```python
from build123d import *

# Parameters (mm, degrees)
MODEL_R             = 1.55
BOSS_EXTRUDE1_DEPTH = 3


with BuildPart() as part:
    # Model → Boss-Extrude1 (new body)
    with BuildSketch(Plane.XY):
        with BuildLine():
            Line((0, 108.6), (0, 5))
            ThreePointArc((0, 5), (1.464466094, 1.464466094), (5, 0))
            Line((5, 0), (365.775, 0))
            ThreePointArc((365.775, 0), (369.310533906, 1.464466094), (370.775, 5))
            Line((370.775, 5), (370.775, 108.6))
            ThreePointArc((370.775, 108.6), (369.310533906, 112.135533906), (365.775, 113.6))
            Line((365.775, 113.6), (5, 113.6))
            ThreePointArc((5, 113.6), (1.464466094, 112.135533906), (0, 108.6))
        make_face()
        with Locations((195.3875, 109.1)):
            Circle(MODEL_R, mode=Mode.SUBTRACT)
        with Locations((175.3875, 109.1)):
            Circle(MODEL_R, mode=Mode.SUBTRACT)
        with Locations((85.3875, 107.6)):
            Circle(MODEL_R, mode=Mode.SUBTRACT)
        with Locations((285.3875, 107.6)):
            Circle(MODEL_R, mode=Mode.SUBTRACT)
        with Locations((85.3875, 6)):
            Circle(MODEL_R, mode=Mode.SUBTRACT)
        with Locations((185.3875, 6)):
            Circle(MODEL_R, mode=Mode.SUBTRACT)
        with Locations((285.3875, 6)):
            Circle(MODEL_R, mode=Mode.SUBTRACT)
        Polygon((9, 9), (361.775, 9), (361.775, 104.6), (190.3875, 104.6), (190.3875, 106.6), (180.3875, 106.6), (180.3875, 104.6), (9, 104.6), align=None, mode=Mode.SUBTRACT)
        Polygon((365.947431604, 110.609548911), (367.784548911, 108.772431604), (367.112117307, 106.262882693), (364.602568396, 105.590451089), (362.765451089, 107.427568396), (363.437882693, 109.937117307), align=None, mode=Mode.SUBTRACT)
        Polygon((4.827568396, 110.609548911), (2.990451089, 108.772431604), (3.662882693, 106.262882693), (6.172431604, 105.590451089), (8.009548911, 107.427568396), (7.337117307, 109.937117307), align=None, mode=Mode.SUBTRACT)
        Polygon((365.947431604, 2.990451089), (367.784548911, 4.827568396), (367.112117307, 7.337117307), (364.602568396, 8.009548911), (362.765451089, 6.172431604), (363.437882693, 3.662882693), align=None, mode=Mode.SUBTRACT)
        Polygon((126.799038106, 2.25), (124.200961894, 2.25), (122.901923789, 4.5), (124.200961894, 6.75), (126.799038106, 6.75), (128.098076211, 4.5), align=None, mode=Mode.SUBTRACT)
        Polygon((4.827568396, 2.990451089), (2.990451089, 4.827568396), (3.662882693, 7.337117307), (6.172431604, 8.009548911), (8.009548911, 6.172431604), (7.337117307, 3.662882693), align=None, mode=Mode.SUBTRACT)
        Polygon((126.799038106, 111.35), (124.200961894, 111.35), (122.901923789, 109.1), (124.200961894, 106.85), (126.799038106, 106.85), (128.098076211, 109.1), align=None, mode=Mode.SUBTRACT)
        Polygon((243.975961894, 2.25), (246.574038106, 2.25), (247.873076211, 4.5), (246.574038106, 6.75), (243.975961894, 6.75), (242.676923789, 4.5), align=None, mode=Mode.SUBTRACT)
        Polygon((243.975961894, 111.35), (246.574038106, 111.35), (247.873076211, 109.1), (246.574038106, 106.85), (243.975961894, 106.85), (242.676923789, 109.1), align=None, mode=Mode.SUBTRACT)
    extrude(amount=BOSS_EXTRUDE1_DEPTH)


solid = part.part
```
Model file for the job. Use its own axes, mm. Coordinates: 2 decimals unless noted, no trailing zeros. Write each loop counter-clockwise with the first axis right and the second up, starting at its lowest first coordinate (ties: lowest second). Pieces come first, ordered by that corner, then holes. Notation, with made-up numbers: (-8.75, 68.25) - (46.25, 68.25) arc R14 cw to (46.25, 77.25) - close; hole circle Ø10 at (28.5, 3). An arc over 180 degrees is marked (long way). One line per item, written item: value. Start each with the question number.
1. Slice it at B-B (z = 0.95). Count the separate pieces of the cut face and the enclosed holes in it, plus the area to 3 significant figures.
2. Probe line 1 (Y direction, x = 126, z = 2.4); line 2 (Y direction, x = 137, z = 1.85); line 3 (X direction, y = 37, z = 0.85) (3 decimals). List the from-to ranges inside material, lowest first. Write a range as from..to.
3. Slice it at A-A (y = 13.5). Write the cut outline in (x, z) (3 decimals).
Answers below:
1. separate pieces: 1
1. enclosed holes: 16
1. area: 8,160 mm^2
2. line 1: y = 0..2.25, 6.75..9, 104.6..106.85, 111.35..113.6
2. line 2: y = 0..9, 104.6..113.6
2. line 3: x = 0..9, 361.775..370.775
3. outline: (0, 0) - (9, 0) - (9, 3) - (0, 3) - close; (361.775, 0) - (370.775, 0) - (370.775, 3) - (361.775, 3) - close
